Geometry: see drawing. Coordinates: mm, zero at the bounding-box minimum. Give positions to 0.01 mm unless a question says otherwise; leave off trailing zeros. Write each loop counter-clockwise with the first axis right and the second up, starting at its lowest first coordinate (ties: lowest second). Pieces come first, ordered by that corner, then holes. Notation, with made-up numbers: M -18.5,74 L -5.5,74 A16 ccw -5.5,102 Z; hole C 53.25,70.25 d5. An arc over 180 degrees is marked long. Use a Markdown table: item, result. Add a question column.
(1) Cut plane A-A (y = 3.5). Output: boundary loops of the cut face in (x, z), plus the area to 3 significant figures.
(2) Cut plane C-C (z = 14). Output: boundary loops of the cut face in (x, y).
(3) Pin query (flat end, axial travel): pin 1 Ø1.5 at (x, y) = (4, 2) entering from +Z. Return the tip coordinate at first contact, or that it passes through.
(4) Material intervals for L1, parallel to Y at x = 3.5, z = 11.5; L2, parallel to X at y = 5, z = 22; L3, parallel to Y at x = 2.75, z = 8.5, sorted ascending.
(5) Draft query along X for the marked faces 1 and 2. Return one class per face: released by +X, released by -X, zero draft, split by the parting line, or undercut.
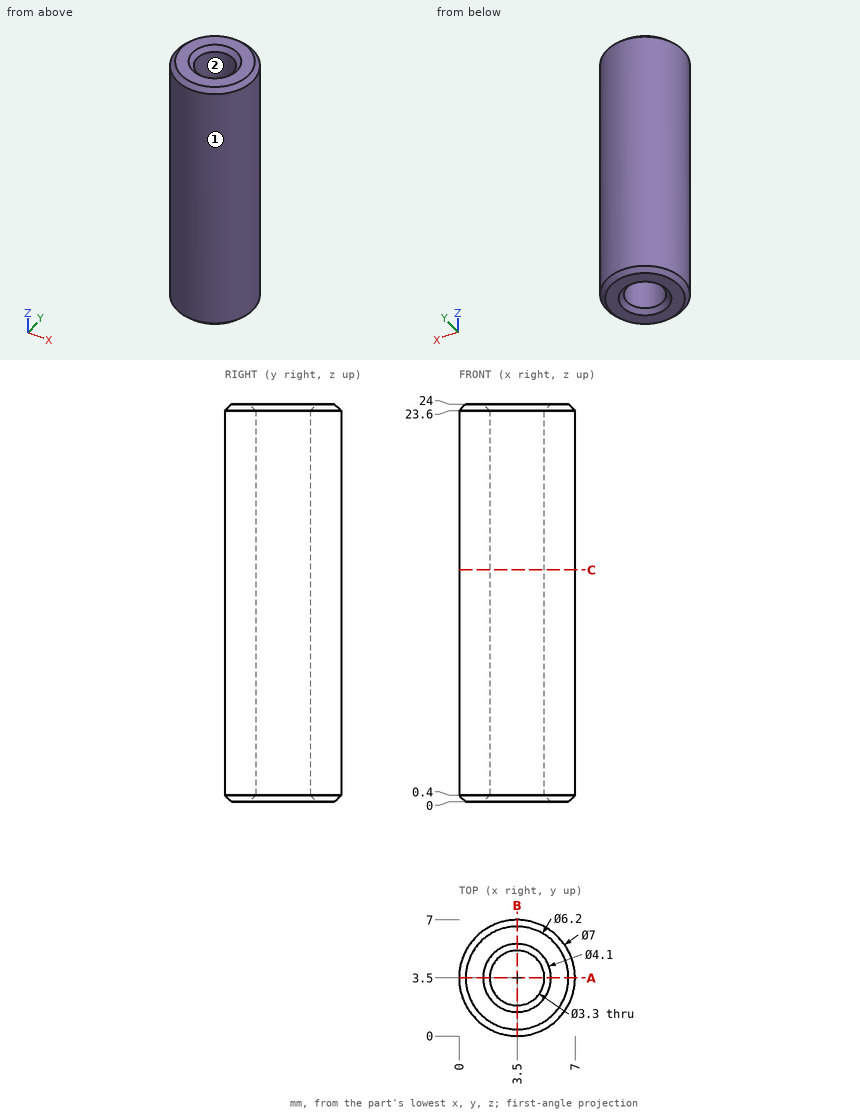
Answer list:
| question | item | result |
|---|---|---|
| 1 | outline | M 0,0.4 L 0.4,0 L 1.45,0 L 1.85,0.4 L 1.85,23.6 L 1.45,24 L 0.4,24 L 0,23.6 Z; M 5.15,0.4 L 5.55,0 L 6.6,0 L 7,0.4 L 7,23.6 L 6.6,24 L 5.55,24 L 5.15,23.6 Z |
| 1 | area | 88.2 mm² |
| 2 | outline | C 3.5,3.5 d7; hole C 3.5,3.5 d3.3 |
| 3 | pin 1 | z = 24 |
| 4 | L1 | 0 to 1.85, 5.15 to 7 |
| 4 | L2 | 0.34 to 2.81, 4.19 to 6.66 |
| 4 | L3 | 0.08 to 2.03, 4.97 to 6.92 |
| 5 | face 1 | split by the parting line |
| 5 | face 2 | undercut |
